```python
from build123d import *

# Parameters (mm, degrees)
F0_W     = 97
F0_H     = 130
F0_W_2   = 93
F0_H_2   = 30
F1_DEPTH = 35
F2_DEPTH = 2


with BuildPart() as f1:
    # F0 (on Top) → F1 (new body)
    with BuildSketch(Plane.XY):
        with Locations((0.344695, -1.031602)):
            Rectangle(F0_W, F0_H)
        with Locations((0.344695, -49.031602)):
            Rectangle(F0_W_2, F0_H_2, mode=Mode.SUBTRACT)
        with Locations((0.344695, -17.031602)):
            Rectangle(F0_W_2, F0_H_2, mode=Mode.SUBTRACT)
        with Locations((0.344695, 14.968398)):
            Rectangle(F0_W_2, F0_H_2, mode=Mode.SUBTRACT)
        with Locations((0.344695, 46.968398)):
            Rectangle(F0_W_2, F0_H_2, mode=Mode.SUBTRACT)
    extrude(amount=F1_DEPTH)

    # F0 (on Top) → F2 (join)
    with BuildSketch(Plane.XY):
        with Locations((0.344695, -49.031602)):
            Rectangle(F0_W_2, F0_H_2)
        with Locations((0.344695, -17.031602)):
            Rectangle(F0_W_2, F0_H_2)
        with Locations((0.344695, 14.968398)):
            Rectangle(F0_W_2, F0_H_2)
        with Locations((0.344695, 46.968398)):
            Rectangle(F0_W_2, F0_H_2)
    extrude(amount=F2_DEPTH)


solid = f1.part
```
The model under review builds one solid part; all positions refer to its coordinate system, in mm. A direction names the side the tool comes from. Coordinates: 2 decimals unless noted, no trailing zeros. Write each loop counter-clockwise with the first axis right and the second up, starting at its lowest first coordinate (ties: lowest second). Pieces come first, ordered by that corner, then holes.
1) We need section A-A on z = 13.5. State the section outline as (x, y) points, then the cut area to 3 significant figures.
2) We need section B-B on y = 9. State the section outline as (x, z) points, then the cut area to 3 significant figures.
3) Clearance check with a flat-ended pin moving along its axis: pin 1 Ø1.5 at (x, y) = (16, 26) entering from +Z. State where the tip first meets the part, or that it passes through.
4) We need section C-C on x = 16. State the section outline as (y, z) points.
5) Machinability: for faces 1 (the face through (48.845, -2, 17)), 2 (the face through (46.845, 15, 18)), which of the approach directions +Z, -Z, +X, -X, +Y, -Y give a long, thin tool a straight path to every point of the face, cutting with its end or side? Answer none if there is none.
6) The part is to be moulded in two halves that separate along X. For faces 3 (the face through (0, 47, 2)), 4 (the face through (0, 63.968, 17)), 5 (the face through (-48.155, -2, 17)), say which applies: pulls with the +X half, pulls with the -X half, needs draft (parallel to the pull), parting line crosses it, or undercut.
7) To check wall thickness, follow probe 1 along Y at (x, z) = (17, 25.5); probe 2 along X at (y, z) = (-43, 4.5); probe 3 along Z at (x, y) = (-3.5, -9.5). State the ranges of each line that lie inside material, in increasing order.
Answer list:
1. outline: (-48.16, -66.03) - (48.84, -66.03) - (48.84, 63.97) - (-48.16, 63.97) - close; hole (-46.16, -64.03) - (46.84, -64.03) - (46.84, -34.03) - (-46.16, -34.03) - close; hole (-46.16, -32.03) - (46.84, -32.03) - (46.84, -2.03) - (-46.16, -2.03) - close; hole (-46.16, -0.03) - (46.84, -0.03) - (46.84, 29.97) - (-46.16, 29.97) - close; hole (-46.16, 31.97) - (46.84, 31.97) - (46.84, 61.97) - (-46.16, 61.97) - close
1. area: 1,450 mm2
2. outline: (-48.16, 0) - (48.84, 0) - (48.84, 35) - (46.84, 35) - (46.84, 2) - (-46.16, 2) - (-46.16, 35) - (-48.16, 35) - close
2. area: 326 mm2
3. pin 1: stops at z = 2
4. outline: (-66.03, 0) - (63.97, 0) - (63.97, 35) - (61.97, 35) - (61.97, 2) - (31.97, 2) - (31.97, 35) - (29.97, 35) - (29.97, 2) - (-0.03, 2) - (-0.03, 35) - (-2.03, 35) - (-2.03, 2) - (-32.03, 2) - (-32.03, 35) - (-34.03, 35) - (-34.03, 2) - (-64.03, 2) - (-64.03, 35) - (-66.03, 35) - close
5. face 1: +Z, -Z, +X, +Y, -Y
5. face 2: +Z
6. face 3: undercut
6. face 4: needs draft
6. face 5: pulls with the -X half
7. probe 1: y = -66.03 to -64.03, -34.03 to -32.03, -2.03 to -0.03, 29.97 to 31.97, 61.97 to 63.97
7. probe 2: x = -48.16 to -46.16, 46.84 to 48.84
7. probe 3: z = 0 to 2
